Work out the finished part from the listing and answer in its coordinate system (mm). Face numbers are marked on the shaded views. A direction names the side the tool comes from. Round coordinates to 2 decimals unless told otherwise and drop trailing zeros. Write each loop counter-clockwise with the first axis right and the second up, starting at its lowest first coordinate (ties: lowest second). Pieces come first, ordered by that corner, then holes. Notation, with made-up numbers: M 53,-19.75 L 83,-19.75 A7 ccw 83,-10.75 Z; hole C -10,49.25 d9. An arc over 180 degrees is marked long. One line per item, written item: value. Start each with the question number.
Q1. Find section C-C (z = -50.5). Write down the section's boundary in (x, y), and give its area (3 significant figures).
Q2. A tool of negligible diameter and unlimited length cuts with its end or side. For the marked faces 3, 4, 5, 6 and 7, from which of +Z, -Z, +X, -X, +Y, -Y can it reach the whole face along a straight path? Write none if from no direction.
Q3. Find section B-B (x = -7.5). Write down the section's boundary in (y, z).
Q4. Find section D-D (x = -42). Write down the section's boundary in (y, z), and give its area (3 significant figures).
Q5. Consider probe 1 along X at (y, z) = (3.5, -35.5); probe 2 along Z at (x, y) = (-12.5, 3.5); probe 3 along Z at (x, y) = (-51, 0.55). Determine where each line is inside the solid, lowest interval first.
Q6. Find section A-A (y = 8.75). Write down the section's boundary in (x, z).
Q7. The mould has two halves that part along X. Classify the marked faces 1 and 2: released by +X, released by -X, zero draft, split by the parting line, or undercut.
Q8. Given pin 1 Ø3 at (y, z) = (6, -18.5) entering from +X; pin 2 Ø1 at (x, y) = (-48.5, 3) entering from -Z; pin 3 Ø5.5 at (y, z) = (9.5, -2) entering from +X, each flat-ended and moving along its own axis, determine where each tip first touches the part or whether it passes through.
Autodesk Inventor part; units mm, degrees
ref_plane "YZ Plane" through (0, 0, 0) normal (1, 0, 0) x (0, 1, 0)
ref_plane "XZ Plane" through (0, 0, 0) normal (0, 1, 0) x (-1, 0, 0)
ref_plane "XY Plane" through (0, 0, 0) normal (0, 0, 1) x (1, 0, 0)
sketch "Эскиз1" plane through (0, 0, 0) normal (0, 1, 0) x (-1, 0, 0)
  line L0 (0, 0) -> (53.5, 0)
  line L1 (53.5, 0) -> (53.5, -66)
  line L2 (53.5, -66) -> (0, -66)
  line L3 (0, -66) -> (0, 0)
  line L4 (53.5, -66) -> (40.5, -66)
  line L5 (40.5, -66) -> (3, -66)
  line L6 (3, -66) -> (3, -68.5)
  line L7 (3, -68.5) -> (40.5, -68.5)
  line L8 (40.5, -68.5) -> (40.5, -66)
  point P0 (3, -66)
  dimension "d0" = 53.5
  dimension "d1" = 66
  dimension "d4" = 13
  dimension "d5" = 37.5
  dimension "d6" = 2.5
extrude "Выдавливание1" add sketch "Эскиз1" along normal blind 1.5
sketch "Эскиз2" plane through (0, 1.5, 0) normal (0, 1, 0) x (1, 0, 0)
  line L0 (-40.5, 66) -> (-53.5, 66)
  line L1 (-53.5, 66) -> (-52, 66)
  line L2 (-52, 66) -> (-52, 65)
  line L3 (-52, 65) -> (-49.7, 65)
  line L4 (-49.7, 65) -> (-49.7, 44)
  line L5 (-49.7, 44) -> (-52, 44)
  line L6 (-52, 44) -> (-52, 65)
  line L7 (-49.7, 44) -> (-49.7, 43)
  line L8 (-49.7, 43) -> (-52, 43)
  line L9 (-52, 43) -> (-52, 17.2)
  line L10 (-52, 17.2) -> (-49.7, 17.2)
  line L11 (-49.7, 17.2) -> (-49.7, 43)
  point P0 (0, 0)
  dimension "d15" = 1.5
  dimension "d16" = 1
  dimension "d17" = 2.3
  dimension "d18" = 21
  dimension "d19" = 1
  dimension "d20" = 25.8
extrude "Выдавливание2" add sketch "Эскиз2" along normal blind 8.5
sketch "Эскиз3" plane through (0, 1.5, 0) normal (0, 1, 0) x (1, 0, 0)
  line L0 (-53.5, 66) -> (-53.5, 0)
  line L1 (-53.5, 0) -> (-53.5, 3)
  line L2 (-53.5, 3) -> (-52.5, 3)
  line L3 (-52.5, 3) -> (-46.5, 3)
  line L4 (-46.5, 3) -> (-46.5, 9.5)
  line L5 (-46.5, 9.5) -> (-52.5, 9.5)
  line L6 (-52.5, 9.5) -> (-52.5, 3)
  point P0 (0, 0)
  dimension "d23" = 3
  dimension "d24" = 1
  dimension "d25" = 6
  dimension "d26" = 6.5
extrude "Выдавливание3" add sketch "Эскиз3" along normal blind 2
sketch "Эскиз4" plane through (0, 3.5, 0) normal (0, 1, 0) x (1, 0, 0)
  line L0 (-52.5, 3) -> (-52.5, 9.5)
  line L1 (-52.5, 6.25) -> (-46.5, 6.25)
  line L2 (-46.5, 3) -> (-46.5, 9.5)
  circle A0 centre (-49.5, 6.25) radius 1.5
  point P0 (0, 0)
  dimension "d29" = 3
extrude "Выдавливание4" add sketch "Эскиз4" along normal blind 0.5
sketch "Эскиз5" plane through (0, 1.5, 0) normal (0, 1, 0) x (1, 0, 0)
  line L0 (-46.5, 9.5) -> (-52.5, 9.5)
  line L1 (-46.5, 9.5) -> (-44.5, 9.5)
  line L2 (-44.5, 9.5) -> (-32.2, 9.5)
  line L3 (-32.2, 9.5) -> (-32.2, -7.1)
  line L4 (-32.2, -7.1) -> (-44.5, -7.1)
  line L5 (-44.5, -7.1) -> (-44.5, 9.5)
  point P0 (0, 0)
  dimension "d32" = 2
  dimension "d33" = 12.3
  dimension "d34" = 16.6
extrude "Выдавливание5" add sketch "Эскиз5" along normal blind 10.8
sketch "Эскиз6" plane through (0, 1.5, 0) normal (0, 1, 0) x (1, 0, 0)
  line L0 (-32.2, 0) -> (0, 0)
  line L1 (0, 0) -> (-4, 0)
  line L2 (-4, 0) -> (-4, 12)
  line L3 (-4, 12) -> (-13, 12)
  line L4 (-13, 12) -> (-13, -2)
  line L5 (-13, -2) -> (-4, -2)
  line L6 (-4, -2) -> (-4, 12)
  dimension "d37" = 4
  dimension "d38" = 12
  dimension "d39" = 9
  dimension "d40" = 14
extrude "Выдавливание6" add sketch "Эскиз6" along normal blind 11
sketch "Эскиз7" plane through (0, 12.5, 0) normal (0, 1, 0) x (1, 0, 0)
  line L0 (-13, 12) -> (-13, -2)
  line L1 (-13, 12) -> (-4, 12)
  line L2 (-4, 12) -> (-4, 1)
  line L3 (-4, 1) -> (-13, 1)
  line L4 (-13, 1) -> (-13, 12)
  point P0 (0, 0)
  dimension "d43" = 11
extrude "Выдавливание7" cut sketch "Эскиз7" against normal blind 1
sketch "Эскиз8" plane through (0, 1.5, 0) normal (0, 1, 0) x (1, 0, 0)
  line L0 (0, 0) -> (0, 66)
  line L1 (0, 66) -> (0, 65)
  line L2 (0, 65) -> (-1.5, 65)
  line L3 (-1.5, 65) -> (-3.8, 65)
  line L4 (-3.8, 65) -> (-3.8, 49)
  line L5 (-3.8, 49) -> (-1.5, 49)
  line L6 (-1.5, 49) -> (-1.5, 65)
  line L7 (-1.5, 49) -> (-1.5, 47)
  line L8 (-1.5, 47) -> (-3.8, 47)
  line L9 (-3.8, 47) -> (-3.8, 26.5)
  line L10 (-3.8, 26.5) -> (-1.5, 26.5)
  line L11 (-1.5, 26.5) -> (-1.5, 47)
  dimension "d47" = 1
  dimension "d48" = 1.5
  dimension "d49" = 2.3
  dimension "d50" = 16
  dimension "d51" = 2
  dimension "d52" = 20.5
extrude "Выдавливание8" add sketch "Эскиз8" along normal blind 8.5
sketch "Эскиз9" plane through (0, 1.5, 0) normal (0, 1, 0) x (1, 0, 0)
  line L0 (0, 0) -> (0, 66)
  line L1 (0, 66) -> (-21.5, 66)
  line L2 (-21.5, 66) -> (-21.5, 26)
  line L3 (-21.5, 26) -> (-11.5, 26)
  line L4 (-11.5, 26) -> (-11.5, 61.5)
  line L5 (-11.5, 61.5) -> (-21.5, 61.5)
  line L6 (-21.5, 61.5) -> (-21.5, 26)
  dimension "d55" = 21.5
  dimension "d56" = 40
  dimension "d57" = 10
  dimension "d58" = 35.5
extrude "Выдавливание9" add sketch "Эскиз9" along normal blind 8
sketch "Эскиз10" plane through (0, 1.5, 0) normal (0, 1, 0) x (1, 0, 0)
  line L0 (-40.5, 68.5) -> (-40.5, 66)
  line L1 (-40.5, 68.5) -> (-36, 68.5)
  line L2 (-3, 68.5) -> (-40.5, 68.5)
  line L3 (-36, 68.5) -> (-36, 66)
  line L4 (-3, 68.5) -> (-7.5, 68.5)
  line L5 (-7.5, 68.5) -> (-7.5, 66)
  line L6 (0, 0) -> (0, 13.5)
  line L7 (0, 0) -> (0, 66)
  line L8 (0, 13.5) -> (-2.5, 13.5)
  line L9 (-53.5, 66) -> (-53.5, 0)
  line L10 (-53.5, 0) -> (-53.5, 15)
  line L11 (-53.5, 15) -> (-51, 15)
  dimension "d67" = 4.5
  dimension "d68" = 2.5
  dimension "d69" = 4.5
  dimension "d70" = 2.5
  dimension "d71" = 13.5
  dimension "d72" = 2.5
  dimension "d73" = 15
  dimension "d74" = 2.5
hole "Отверстие1" at (-51, 1.5, -15) at (-2.5, 1.5, -13.5) at (-7.5, 1.5, -66) at (-36, 1.5, -66) direction (0, -1, 0) diameter 3 end through all
chamfer "Фаска3" distance 2.5 angle 45 2 edges at (-40.5, 0.75, -68.5) (-3, 0.75, -68.5)
chamfer "Фаска4" distance 1 angle 45 1 edges at (-53.5, 0.75, -66)
properties part number "Arduino UNO"
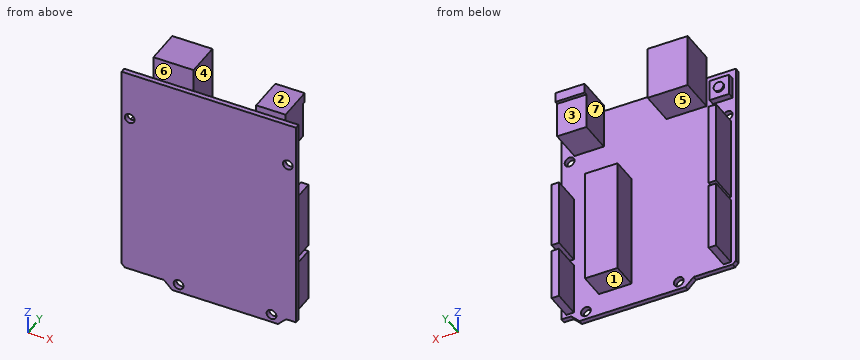
The answers:
1. outline: M -53.5,0 L 0,0 L 0,1.5 L -1.5,1.5 L -1.5,10 L -3.8,10 L -3.8,1.5 L -11.5,1.5 L -11.5,9.5 L -21.5,9.5 L -21.5,1.5 L -49.7,1.5 L -49.7,10 L -52,10 L -52,1.5 L -53.5,1.5 Z
1. area: 199 mm2
2. face 3: -Z, +X, +Y
2. face 4: +Z, -Z, +Y
2. face 5: -Z, -X, +Y
2. face 6: +Z, +X, -X, -Y
2. face 7: +Z, +Y
3. outline: M 0,-68.5 L 1.5,-68.5 L 1.5,-67.5 L 0,-67.5 Z; M 0,-64.5 L 1.5,-64.5 L 1.5,-12 L 11.5,-12 L 11.5,-1 L 12.5,-1 L 12.5,2 L 1.5,2 L 1.5,0 L 0,0 Z
4. outline: M 0,-66 L 1.5,-66 L 1.5,-9.5 L 12.3,-9.5 L 12.3,7.1 L 1.5,7.1 L 1.5,0 L 0,0 Z
4. area: 278 mm2
5. probe 1: -52 to -49.7, -21.5 to -11.5, -3.8 to -1.5
5. probe 2: -61.5 to -26, -12 to 2
5. probe 3: -66 to -16.5, -13.5 to 0
6. outline: M -52,-65 L -49.7,-65 L -49.7,-44 L -52,-44 Z; M -52,-43 L -49.7,-43 L -49.7,-17.2 L -52,-17.2 Z; M -44.5,-9.5 L -32.2,-9.5 L -32.2,7.1 L -44.5,7.1 Z; M -21.5,-61.5 L -11.5,-61.5 L -11.5,-26 L -21.5,-26 Z; M -13,-12 L -4,-12 L -4,2 L -13,2 Z; M -3.8,-65 L -1.5,-65 L -1.5,-49 L -3.8,-49 Z; M -3.8,-47 L -1.5,-47 L -1.5,-26.5 L -3.8,-26.5 Z
7. face 1: undercut
7. face 2: zero draft
8. pin 1: x = -49.7
8. pin 2: z = -9.5
8. pin 3: x = -4
